Source: CAD feature listing. Evaluate the final solid. Frame: model axes, mm. Coordinates: 2 decimals unless noted, no trailing zeros. Loops run counter-clockwise (first coordinate to the right, second up) from the corner with the lowest first, then second, coordinate; pieces in that order, holes last. Notation, with made-up numbers: (59, -18.75) - (100, -18.75) arc R16 cw to (100, 10.25) - close; hole circle Ø10 at (-30.5, 18). An arc over 180 degrees is marked (long way). Write item = value, one per line. Start each with the question number.
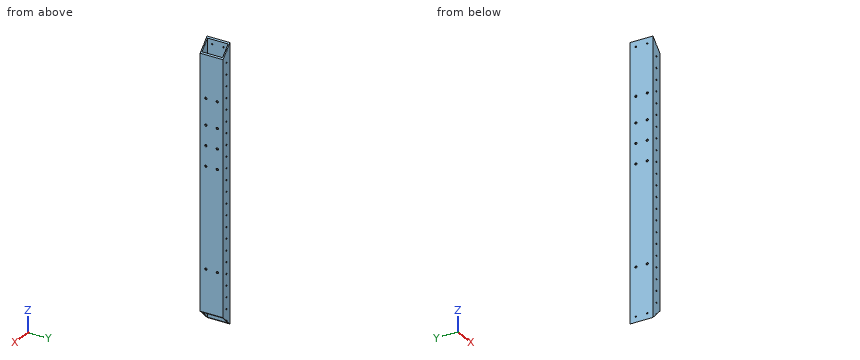
from build123d import *

# Parameters (mm, degrees)
SKETCH1_W           = 25.4
SKETCH1_H           = 50.8
SKETCH1_W_2         = 20.32
SKETCH1_H_2         = 45.72
EXTRUDE_THIN1_DEPTH = 609.6
SKETCH2_R           = 1.5875
CUT_EXTRUDE1_DEPTH  = 51.8
LPATTERN1_COUNT     = 50
LPATTERN1_PITCH     = 25.4
CUT_EXTRUDE2_DEPTH  = 51.8
SKETCH5_R           = 1.5875
CUT_EXTRUDE3_DEPTH  = 26.4
SKETCH7_R           = 2.4892
CUT_EXTRUDE4_DEPTH  = 26.4


with BuildPart() as part:
    # Sketch1 → Extrude-Thin1 (new body)
    with BuildSketch(Plane.XY):
        with Locations((12.7, 25.4)):
            Rectangle(SKETCH1_W, SKETCH1_H)
        with Locations((12.7, 25.4)):
            Rectangle(SKETCH1_W_2, SKETCH1_H_2, mode=Mode.SUBTRACT)
    extrude(amount=EXTRUDE_THIN1_DEPTH)

    # Sketch2 → Cut-Extrude1 (cut, through all)
    with BuildSketch(Plane(origin=(0, 50.8, 0), x_dir=(1, 0, 0), z_dir=(0, 1, 0))):
        with Locations((12.7, -596.9)):
            Circle(SKETCH2_R)
    cut_extrude1 = extrude(amount=-CUT_EXTRUDE1_DEPTH, mode=Mode.SUBTRACT)

    # LPattern1: Cut-Extrude1 ×50
    with Locations(*[(0, 0, -i * LPATTERN1_PITCH) for i in range(1, LPATTERN1_COUNT)]):
        add(cut_extrude1, mode=Mode.SUBTRACT)

    # Sketch4 → Cut-Extrude2 (cut, through all)
    with BuildSketch(Plane(origin=(0, 50.8, 0), x_dir=(1, 0, 0), z_dir=(0, 1, 0))):
        Polygon((0, -609.6), (25.4, -584.2), (25.4, -609.6), align=None)
        Polygon((0, 0), (25.4, 0), (25.4, -25.4), align=None)
    extrude(amount=-CUT_EXTRUDE2_DEPTH, mode=Mode.SUBTRACT)

    # Sketch5 → Cut-Extrude3 (cut, through all)
    with BuildSketch(Plane.ZY):
        with Locations((12.7, 12.7)):
            Circle(SKETCH5_R)
        with Locations((12.7, 38.1)):
            Circle(SKETCH5_R)
        with Locations((596.9, 38.1)):
            Circle(SKETCH5_R)
        with Locations((596.9, 12.7)):
            Circle(SKETCH5_R)
    extrude(amount=-CUT_EXTRUDE3_DEPTH, mode=Mode.SUBTRACT)

    # Sketch7 → Cut-Extrude4 (cut, through all)
    with BuildSketch(Plane.ZY):
        with Locations((489.585, 38.1)):
            Circle(SKETCH7_R)
        with Locations((489.845193373, 12.7)):
            Circle(SKETCH7_R)
        with Locations((120.015, 12.7)):
            Circle(SKETCH7_R)
        with Locations((119.754806627, 38.1)):
            Circle(SKETCH7_R)
        with Locations((342.9, 38.1)):
            Circle(SKETCH7_R)
        with Locations((342.9, 12.7)):
            Circle(SKETCH7_R)
        with Locations((387.35, 12.7)):
            Circle(SKETCH7_R)
        with Locations((387.35, 38.1)):
            Circle(SKETCH7_R)
        with Locations((431.8, 38.1)):
            Circle(SKETCH7_R)
        with Locations((431.8, 12.7)):
            Circle(SKETCH7_R)
    extrude(amount=-CUT_EXTRUDE4_DEPTH, mode=Mode.SUBTRACT)


solid = part.part
Item 1: Cut plane B-B (y = 28). Return the cut outline in (x, z).
Item 2: First-contact query: pin 1 (5 mm diameter, centred on x = 12.7, z = 571.5, fed in from +Y). Flat tip, straight axial feed; report the tip coordinate or a pass-through.
Item 3: Material intervals for L1, parallel to Y at x = 24.55, z = 387.35; L2, parallel to Y at x = 20, z = 464; L3, parallel to X at y = 20, z = 344, sorted ascending. Write a range as [from, to].
Item 4: Cut plane A-A (z = 75). Return the cut outline in (x, y), then the cut area to 3 significant figures.
Responses:
q1.outline = (0, 0) - (2.54, 2.54) - (2.54, 607.06) - (0, 609.6) - close; (22.86, 22.86) - (25.4, 25.4) - (25.4, 584.2) - (22.86, 586.74) - close
q2.pin_1 = 50.8
q3.L1 = [0, 10.21], [15.19, 35.61], [40.59, 50.8]
q3.L2 = [0, 2.54], [48.26, 50.8]
q3.L3 = [0, 2.54], [22.86, 25.4]
q4.outline = (0, 0) - (25.4, 0) - (25.4, 50.8) - (0, 50.8) - close; hole (2.54, 2.54) - (22.86, 2.54) - (22.86, 48.26) - (2.54, 48.26) - close
q4.area = 361 mm2
